The drawing under review shows one solid part. Ordinate dimensions are in mm from its lowest x, y, z. Round coordinates to 2 decimals unless told otherwise and drop trailing zeros. Order: outer loops, then holes, each group sorted by start corner. A loop starts at its lowest first (then second) coordinate and runs counter-clockwise, first axis right, second up. Notation, with made-up numbers: M 26,-33 L 62,-33 A15 ccw 62,-23 Z; hole C 25.5,16.5 d3. An arc over 180 degrees is marked long. Answer as a JSON object with one key per item and string values. Group by question number.
1) Consider section B-B, the plane z = 0.4. Write out the cut boundary in (x, y), then the cut area to 3 significant figures.
2) To check wall thickness, follow line 1 (Z direction, x = 1, y = 0.2); line 2 (X direction, y = 0.1, z = 1.25). State the ranges of each line that lie inside material, in increasing order.
3) Consider section A-A, the plane y = 0.35. Write out the cut boundary in (x, z).
4) Consider section C-C, the plane x = 8.25. Write out the cut boundary in (y, z), then the cut area to 3 significant figures.
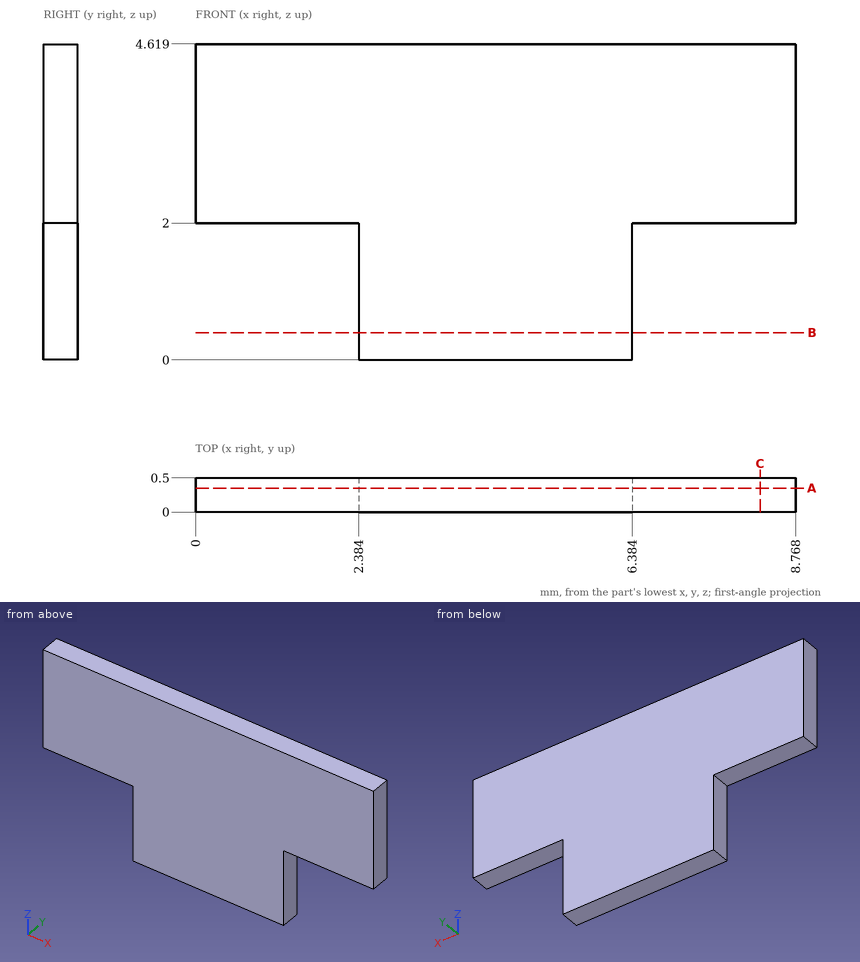
Results list:
{
 "1": {"outline": "M 2.38,0 L 6.38,0 L 6.38,0.5 L 2.38,0.5 Z", "area": "2.00 mm^2"},
 "2": {"line 1": "2 to 4.62", "line 2": "2.38 to 6.38"},
 "3": {"outline": "M 0,2 L 2.38,2 L 2.38,0 L 6.38,0 L 6.38,2 L 8.77,2 L 8.77,4.62 L 0,4.62 Z"},
 "4": {"outline": "M 0,2 L 0.5,2 L 0.5,4.62 L 0,4.62 Z", "area": "1.31 mm^2"}
}
